```python
from build123d import *

# Parameters (mm, degrees)
F0_W     = 1.5875
F0_H     = 4.7625
F1_DEPTH = 24.13
F0_W_2   = 19.05
F2_DEPTH = 3.175
F3_R     = 0.79375
F4_DEPTH = 8.89
F5_R     = 0.79375
F6_DEPTH = 8.89


with BuildPart() as f1:
    # F0 (on Top) → F1 (new body)
    with BuildSketch(Plane.XY):
        with Locations((-10.31875, 0)):
            Rectangle(F0_W, F0_H)
    extrude(amount=F1_DEPTH)



with BuildPart() as f1b:
    # F0 (on Top) → F1, piece 2 (new body)
    with BuildSketch(Plane.XY):
        with Locations((10.31875, 0)):
            Rectangle(F0_W, F0_H)
    extrude(amount=F1_DEPTH)


with BuildPart() as f1_1:
    add(f1.part)

    add(f1b.part)  # F2 merges F1b
    # F0 (on Top) → F2 (join)
    with BuildSketch(Plane.XY):
        with Locations((-10.31875, 0)):
            Rectangle(F0_W, F0_H)
        Rectangle(F0_W_2, F0_H)
        with Locations((10.31875, 0)):
            Rectangle(F0_W, F0_H)
    extrude(amount=F2_DEPTH)

    # F3 (on face) → F4 (join)
    with BuildSketch(Plane.YZ.offset(11.1125)):
        with Locations((0, 11.1125)):
            Circle(F3_R)
        with Locations((0, 20.6375)):
            Circle(F3_R)
    extrude(amount=-F4_DEPTH)

    # F5 (on face) → F6 (join)
    with BuildSketch(Plane(origin=(-11.1125, 0, 0), x_dir=(0, -1, 0), z_dir=(-1, 0, 0))):
        with Locations((0, 11.1125)):
            Circle(F5_R)
        with Locations((0, 20.6375)):
            Circle(F5_R)
    extrude(amount=-F6_DEPTH)


solid = f1_1.part
```
For this review, take the finished solid that the model builds, in its own axes (mm). A direction names the side the tool comes from. Coordinates: 2 decimals unless noted, no trailing zeros. Loops run counter-clockwise (first coordinate to the right, second up) from the corner with the lowest first, then second, coordinate; pieces in that order, holes last. Notation, with made-up numbers: (2.25, 34.25) -> (60.25, 34.25) arc R18 cw to (60.25, 44.25) -> close; hole circle Ø8 at (4, -1.5). An arc over 180 degrees is marked (long way). Return JSON: item names as keys, results as strings. Group by question number.
(1) Consider section D-D, the plane x = 0.5. Give the boundary of the cut face in (y, z) (3 decimals), plus the area to 3 significant figures.
(2) To check wall thickness, follow L1, parallel to X at y = 0.6, z = 18.5 (1 decimal); L2, parallel to Z at x = -2.5, y = 0.7 (3 decimals); L3, parallel to Z at x = -6.25, y = 1.75 (3 decimals). State the ranges of each line that lie inside material, in increasing order.
(3) For pin 1 Ø3 at (x, z) = (-4.5, 20.5) entering from +Y; pin 2 Ø8 at (x, z) = (-4, 5.5) entering from -Y, all flat-tipped, find the tip position at first contact; note any pin that passes through.
(4) Consider section C-C, the plane x = 6.25. Give the boundary of the cut face in (y, z) (1 decimal), plus the area to 3 significant figures.
(5) Tool access review of faces 4 (the flat face through (-2.222, 0, 11)), 5 (the flat face through (0, 0, 3.175)), 6 (the cylindrical face through (-5.9, -0.4, 11.8)), 7 (the flat face through (0, -2.381, 3)), 8 (the flat face through (0, 0, 0)): name each direction out of +Z, -Z, +X, -X, +Y, -Y from which nothing blocks a thin tool from reaching the whole face with its end or side.
(6) Consider section A-A, the plane z = 6.25. Give the boundary of the cut face in (x, y) (1 decimal), plus the area to 3 significant figures.
(7) Mouldability with a two-part tool opening along X and no side actions: class faces 1 (the flat face through (10, 0, 24.13)), 2 (the flat face through (11.112, 0, 12)), 3 (the flat face through (9.525, 0, 14)) as pulls with the +X half, pulls with the -X half, needs draft (parallel to the pull), parting line crosses it, or undercut.
(8) Consider section B-B, the plane y = 0. Give the boundary of the cut face in (x, z) (1 decimal), plus the area to 3 significant figures.
Results below:
{
 "1": {"outline": "(-2.381, 0) -> (2.381, 0) -> (2.381, 3.175) -> (-2.381, 3.175) -> close", "area": "15.1 mm2"},
 "2": {"L1": "x = -11.1 to -9.5, 9.5 to 11.1", "L2": "z = 0 to 3.175, 10.738 to 11.487, 20.263 to 21.012", "L3": "z = 0 to 3.175"},
 "3": {"pin 1": "stops at y = 0.79", "pin 2": "stops at y = -2.38"},
 "4": {"outline": "(-2.4, 0) -> (2.4, 0) -> (2.4, 3.2) -> (-2.4, 3.2) -> close; circle Ø1.6 at (0, 11.1); circle Ø1.6 at (0, 20.6)", "area": "19.1 mm2"},
 "5": {"face 4": "+Z, +Y, -Y", "face 5": "+Y, -Y", "face 6": "none", "face 7": "+Z, -Z, +X, -X, -Y", "face 8": "-Z, +X, -X, +Y, -Y"},
 "6": {"outline": "(-11.1, -2.4) -> (-9.5, -2.4) -> (-9.5, 2.4) -> (-11.1, 2.4) -> close; (9.5, -2.4) -> (11.1, -2.4) -> (11.1, 2.4) -> (9.5, 2.4) -> close", "area": "15.1 mm2"},
 "7": {"face 1": "needs draft", "face 2": "pulls with the +X half", "face 3": "undercut"},
 "8": {"outline": "(-11.1, 0) -> (11.1, 0) -> (11.1, 24.1) -> (9.5, 24.1) -> (9.5, 21.4) -> (2.2, 21.4) -> (2.2, 19.8) -> (9.5, 19.8) -> (9.5, 11.9) -> (2.2, 11.9) -> (2.2, 10.3) -> (9.5, 10.3) -> (9.5, 3.2) -> (-9.5, 3.2) -> (-9.5, 10.3) -> (-2.2, 10.3) -> (-2.2, 11.9) -> (-9.5, 11.9) -> (-9.5, 19.8) -> (-2.2, 19.8) -> (-2.2, 21.4) -> (-9.5, 21.4) -> (-9.5, 24.1) -> (-11.1, 24.1) -> close", "area": "183 mm2"}
}
